from build123d import *

# Parameters (mm, degrees)
SKETCH1_W           = 70
SKETCH1_H           = 40
BOSS_EXTRUDE1_DEPTH = 30
SKETCH2_W           = 30
SKETCH2_H           = 15
CUT_EXTRUDE1_DEPTH  = 31
SKETCH3_W           = 45
SKETCH3_H           = 15
CUT_EXTRUDE2_DEPTH  = 41
SKETCH4_W           = 15.133947596
SKETCH4_H           = 40
BOSS_EXTRUDE2_DEPTH = 15
SKETCH6_R           = 5
CUT_EXTRUDE3_DEPTH  = 16
SKETCH7_R           = 5
CUT_EXTRUDE4_DEPTH  = 16
SKETCH8_W           = 3.137431518
SKETCH8_H           = 25
CUT_EXTRUDE5_DEPTH  = 15


with BuildPart() as part:
    # Sketch1 → Boss-Extrude1 (new body)
    with BuildSketch(Plane(origin=(0, 0, 0), x_dir=(1, 0, 0), z_dir=(0, 1, 0))):
        with Locations((35, 20)):
            Rectangle(SKETCH1_W, SKETCH1_H)
    extrude(amount=BOSS_EXTRUDE1_DEPTH)

    # Sketch2 → Cut-Extrude1 (cut, through all)
    with BuildSketch(Plane(origin=(0, 30, 0), x_dir=(1, 0, 0), z_dir=(0, 1, 0))):
        with Locations((55, 7.5)):
            Rectangle(SKETCH2_W, SKETCH2_H)
    extrude(amount=-CUT_EXTRUDE1_DEPTH, mode=Mode.SUBTRACT)

    # Sketch3 → Cut-Extrude2 (cut, through all)
    with BuildSketch(Plane(origin=(0, 0, -40), x_dir=(-1, 0, 0), z_dir=(0, 0, -1))):
        with Locations((-34.362568482, 22.5)):
            Rectangle(SKETCH3_W, SKETCH3_H)
    extrude(amount=-CUT_EXTRUDE2_DEPTH, mode=Mode.SUBTRACT)

    # Sketch4 → Boss-Extrude2 (add)
    with BuildSketch(Plane(origin=(0, 30, 0), x_dir=(1, 0, 0), z_dir=(0, 1, 0))):
        with Locations((7.566973798, 20)):
            Rectangle(SKETCH4_W, SKETCH4_H)
    extrude(amount=-BOSS_EXTRUDE2_DEPTH)

    # Sketch6 → Cut-Extrude3 (cut, through all)
    with BuildSketch(Plane(origin=(0, 15, 0), x_dir=(1, 0, 0), z_dir=(0, 1, 0))):
        with Locations((40, 30)):
            Circle(SKETCH6_R)
    extrude(amount=-CUT_EXTRUDE3_DEPTH, mode=Mode.SUBTRACT)

    # Sketch7 → Cut-Extrude4 (cut, through all)
    with BuildSketch(Plane(origin=(0, 15, 0), x_dir=(1, 0, 0), z_dir=(0, 1, 0))):
        with Locations((25.133947596, 12.5)):
            Circle(SKETCH7_R)
    extrude(amount=-CUT_EXTRUDE4_DEPTH, mode=Mode.SUBTRACT)

    # Sketch8 → Cut-Extrude5 (cut)
    with BuildSketch(Plane(origin=(0, 30, 0), x_dir=(1, 0, 0), z_dir=(0, 1, 0))):
        with Locations((58.431284241, 27.5)):
            Rectangle(SKETCH8_W, SKETCH8_H)
    extrude(amount=-CUT_EXTRUDE5_DEPTH, mode=Mode.SUBTRACT)


solid = part.part
Can you work these out from the model? Positions are in its coordinate system, mm. A direction names the side the tool comes from. Coordinates: 2 decimals unless noted, no trailing zeros. Write each loop counter-clockwise with the first axis right and the second up, starting at its lowest first coordinate (ties: lowest second). Pieces come first, ordered by that corner, then holes. Notation, with made-up numbers: (73, 67) -> (103, 67) arc R25 cw to (103, 102) -> close; hole circle Ø3 at (37.5, 53.25). An arc over 180 degrees is marked (long way). Write each question's results on one line, items separated by ' | '. Start each with the question number.
Q1. I'm going to push flat-ended pins straight in: pin 1 (8 mm diameter, centred on x = 40, z = -30, fed in from -Y); pin 2 (7.5 mm diameter, centred on y = 5, z = -6, fed in from +X); pin 3 (8 mm diameter, centred on x = 44, y = 16, fed in from +Z). Where does each tip first touch, or does it pass through?
Q2. On a 3-axis mill with a long thin cutter (end or side, diameter ignored), from which of +Z, -Z, +X, -X, +Y, -Y can I reach the whole of each face in a straight line? I mean faces 1 (the face through (60, 23, -27)), 2 (the face through (58, 12, -15)), 3 (the face through (35, 0, -25)). Say none if no direction works.
Q3. We'd pull the mould along Z, two halves only. Please class faces 4 (the face through (35, 8, -30)), 5 (the face through (70, 15, -27)), 6 (the face through (35, 11, -40)), 7 (the face through (15, 11, 0)): +Z half, -Z half, draft (parallel to the pull), parting line (faces both ways), or undercut.
Q4. Imagine slicing it at B-B (y = 5.75). Write out the boundary of the cut face in (x, z).
Q5. Imagine slicing it at C-C (y = 17.5). Write out the boundary of the cut face in (x, z).
Q6. If I drill on probe 1 along X at (y, z) = (27.75, -28.5); probe 2 along X at (y, z) = (5.5, -30); probe 3 along Z at (x, y) = (47, 4.25), over which ranges is the centre line in solid material (lowest first)?
Q7. Imagine slicing it at A-A (z = -30). Write out the boundary of the cut face in (x, y), then the cut area to 3 significant figures.
Q8. Imagine slicing it at D-D (x = 42). Write out the boundary of the cut face in (y, z).
Taken from the geometry:
1) pin 1: passes through | pin 2: stops at x = 40 | pin 3: stops at z = -15
2) face 1: +Z, -Z, +Y | face 2: +Z, +X, +Y, -Y | face 3: +Z, -Z, +X, -X, -Y
3) face 4: undercut | face 5: draft | face 6: -Z half | face 7: +Z half
4) outline: (0, -40) -> (70, -40) -> (70, -15) -> (40, -15) -> (40, 0) -> (0, 0) -> close; hole circle Ø10 at (25.13, -12.5); hole circle Ø10 at (40, -30)
5) outline: (0, -40) -> (15.13, -40) -> (15.13, 0) -> (0, 0) -> close; (60, -40) -> (70, -40) -> (70, -15) -> (60, -15) -> close
6) probe 1: x = 0 to 15.13, 60 to 70 | probe 2: x = 0 to 35, 45 to 70 | probe 3: z = -40 to -15
7) outline: (0, 0) -> (35, 0) -> (35, 15) -> (15.13, 15) -> (15.13, 30) -> (0, 30) -> close; (45, 0) -> (70, 0) -> (70, 30) -> (60, 30) -> (60, 15) -> (45, 15) -> close | area: 1,280 mm^2
8) outline: (0, -40) -> (15, -40) -> (15, -34.58) -> (0, -34.58) -> close; (0, -25.42) -> (15, -25.42) -> (15, -15) -> (0, -15) -> close
